Autodesk Inventor part; units mm, degrees
ref_plane "YZ Plane" through (0, 0, 0) normal (1, 0, 0) x (0, 1, 0)
ref_plane "XZ Plane" through (0, 0, 0) normal (0, 1, 0) x (-1, 0, 0)
ref_plane "XY Plane" through (0, 0, 0) normal (0, 0, 1) x (1, 0, 0)
sketch "Sketch1" plane through (0, 0, 0) normal (0, 1, 0) x (-1, 0, 0)
  circle A0 centre (0, 0) radius 3.175
  circle A1 centre (0, 0) radius 2.54
  dimension "d0" = 6.35
  dimension "d1" = 5.08
extrude "Extrusion1" add sketch "Sketch1" along normal blind 127
sketch "Sketch7" plane through (0, 127, 0) normal (0, 1, 0) x (1, 0, 0)
  circle A0 centre (0, 0) radius 2.54
  circle A1 centre (0, 0) radius 3.175
sketch "Sketch15" plane through (0, 0, 0) normal (1, 0, 0) x (0, 1, 0)
  line L0 (127, -3.175) -> (127, 3.175)
  line L1 (153.67, 7.62) -> (209.55, 7.62)
  line L2 (222.25, 0) -> (209.55, 7.62)
  line L3 (153.67, 7.62) -> (127, 0)
  point P0 (0, 0)
  dimension "d42" = 55.88
sweep "Sweep7" add profiles "Sketch7" path "Sketch15" path curves L3 L1 L2
properties part number "waterpipe"
Design review of the part built by this model. Coordinates are the model's own, in mm. A direction names the side the tool comes from. Give positions to 0.01 mm unless a question says otherwise; leave off trailing zeros. Order: outer loops, then holes, each group sorted by start corner. A loop starts at its lowest first (then second) coordinate and runs counter-clockwise, first axis right, second up. Notation, with made-up numbers: (40.25, -32) - (44.25, -32) arc R9 ccw to (44.25, -23) - close; hole circle Ø10 at (49, 72.25). An arc over 180 degrees is marked (long way). Use a Markdown table: item, result. Add a question column.
(1) Wall thickness on probe 1 along X at (y, z) = (169, 7.5); probe 2 along Z at (x, y) = (0.25, 122); probe 3 along Z at (x, y) = (0, 197.5) (3 decimals): over which ranges is each line inside the solid? List them lowest first. Write a range as [from, to].
(2) Machinability: for faces 1 (the face through (0.69, 62.61, 3.1)), 2 (the face through (0, 0, 3)), which of the approach directions +Z, -Z, +X, -X, +Y, -Y give a long, thin tool a straight path to every point of the face, cutting with its end or side? Answer none if there is none.
(3) Add section A-A on y = 68. Give the boundary of the cut face in (x, z) (3 decimals), then the cut area to 3 significant figures.
(4) Clearance check with flat-ended pins moving along their axes: P1, Ø1, axis at x = 1, y = 185.5, coming from the -Z side; P2, Ø1.5, axis at y = 90.5, z = 4, coming from the -X side; P3, Ø3, axis at x = -2, y = 167, coming from the +Z side. State where each tip first meets the part, or that it passes through.
(5) Mouldability with a two-part tool opening along X and no side actions: class faces 3 (the face through (-0.69, 181.22, 4.52)), 4 (the face through (-0.55, 181.22, 5.14)), 5 (the face through (3, 222.25, 0)) as +X half, -X half, draft (parallel to the pull), parting line (faces both ways), or undercut.
Report:
| question | item | result |
|---|---|---|
| 1 | probe 1 | x = [-3.17, -2.54], [2.54, 3.17] |
| 1 | probe 2 | z = [-3.17, -2.53], [2.53, 3.17] |
| 1 | probe 3 | z = [4.445, 5.08], [10.16, 10.795] |
| 2 | face 1 | -Y |
| 2 | face 2 | +Z, -Z, +X, -X, -Y |
| 3 | outline | circle Ø6.35 at (0, 0); hole circle Ø5.08 at (0, 0) |
| 3 | area | 11.4 mm² |
| 4 | P1 | stops at z = 4.48 |
| 4 | P2 | passes through |
| 4 | P3 | stops at z = 10.76 |
| 5 | face 3 | parting line |
| 5 | face 4 | undercut |
| 5 | face 5 | draft |
